Autodesk Inventor part; units mm, degrees
ref_plane "Work Plane1" through (-4, 0, 0) normal (1, 0, 0) x (0, 1, 0)
ref_plane "XZ Plane" through (0, 0, 0) normal (0, 1, 0) x (-1, 0, 0)
ref_plane "XY Plane" through (0, 0, 0) normal (0, 0, 1) x (1, 0, 0)
sketch "Sketch2" plane through (0, 0, 0) normal (0, 1, 0) x (-1, 0, 0)
  line L0 (-8, -4) -> (8, -4)
  line L1 (-8, 4) -> (8, 4)
  line L2 (-8, -4) -> (-8, 4)
  line L3 (8, 4) -> (8, -4)
  point P0 (0, 0)
  point P1 (0, 4)
  point P2 (-8, 0)
  dimension "d58" = 16
  dimension "d59" = 8
extrude "Extrusion1" add sketch "Sketch2" along normal blind 9.6
sketch "Sketch9" plane through (0, 0, 0) normal (0, -1, 0) x (1, 0, 0)
  line L0 (-8, 4) -> (8, 4)
  line L1 (-8, -4) -> (-8, 4)
  line L2 (-6.5, 2.5) -> (6.5, 2.5)
  line L3 (6.5, 2.5) -> (6.5, -2.5)
  line L4 (6.5, -2.5) -> (-6.5, -2.5)
  line L5 (-6.5, -2.5) -> (-6.5, 2.5)
  point P0 (0, 0)
  point P1 (0, 2.5)
  point P2 (-6.5, 0)
  dimension "d61" = 1.5
  dimension "d62" = 1.5
extrude "Extrusion4" cut sketch "Sketch9" against normal blind 8
sketch "Sketch11" plane through (-8, 0, 4) normal (0, 0, 1) x (1, 0, 0)
  line L0 (0, 0) -> (16, 0)
  line L1 (0, 9.6) -> (16, 9.6)
  line L2 (0, 0) -> (0, 9.6)
  line L3 (7.6, 8) -> (0.4, 8)
  line L4 (0.4, 8) -> (0.4, 5.6)
  arc A0 (0.4, 5.6) -> (7.6, 5.6) centre (4, 5.6) ccw
  line L5 (7.6, 5.6) -> (7.6, 8)
  point P0 (8, 0)
  point P1 (8, 9.6)
  dimension "d93" = 1.6
  dimension "d94" = 4
  dimension "d96" = 7.2
  dimension "d97" = 5.6
extrude "Extrusion5" add sketch "Sketch11" against normal blind 8
sketch "Sketch4" plane through (0, 9.6, 0) normal (0, 1, 0) x (1, 0, 0)
  circle A0 centre (-4, 0) radius 2.4
  circle A1 centre (-4, 0) radius 1.6
  line L0 (-8, 4) -> (-8, -4)
  point P0 (-8, 0)
  dimension "d13" = 4.8
  dimension "d57" = 3.2
  dimension "d69" = 4
extrude "Extrusion3" add sketch "Sketch4" along normal blind 1.6
sketch3d "Sketch12"
feature "LEGO_SM:1" [suppressed]
fillet "Fillet1" radius 0.1 1 edges at (-6.4, 11.2, 0)
pattern_linear "Rectangular Pattern2" count 2 spacing 8 along (1, 0, 0) of "Extrusion3", "Fillet1", "Extrusion5"
fillet "Fillet2" radius 0.1 8 edges at (-8, 9.6, 0) (-8, 4.8, 4) (0, 9.6, 4) (-8, 4.8, -4) (0, 9.6, -4) (8, 4.8, 4) (8, 9.6, 0) (8, 4.8, -4)
ref_plane "Work Plane1" through (-4, 0, 0) normal (1, 0, 0) x (0, 1, 0)
sketch "Sketch10" plane through (-4, 0, 0) normal (1, 0, 0) x (0, 1, 0)
  line L0 (0, -3.9) -> (0, 3.9)
  line L1 (0, 4) -> (9.5, 4)
  line L2 (9.5, -4) -> (0, -4)
  line L3 (5.6, 4) -> (5.6, -4)
  line L4 (5.6, -4) -> (8.8, -4)
  line L5 (8.8, -4) -> (8.8, -3.2)
  line L6 (8.8, -3.2) -> (8, -3.2)
  line L7 (8, -3.2) -> (8, 3.2)
  line L8 (8, 3.2) -> (8.8, 3.2)
  line L9 (8.8, 3.2) -> (8.8, 4)
  line L10 (8.8, 4) -> (5.6, 4)
  line L11 (8.8, 4) -> (9.5, 4)
  line L12 (9.5, -4) -> (8.8, -4)
  line L13 (9.5, -4) -> (9.5, 4)
  point P0 (0, 0)
  dimension "d75" = 5.6
  dimension "d76" = 0.8
  dimension "d77" = 4.8
  dimension "d78" = 6.4
revolve "Revolution1" cut sketch "Sketch10" angle 360 about axis through (-4, 5.6, 4) along (0, 0, -1) contours L1 L9 L8 L7 L6 L5 L2 L3
pattern_linear "Rectangular Pattern4" count 2 spacing 8 along (1, 0, 0) of "Revolution1"
equation "\"d58\" = 0.8 * knobs"
equation "\"d4\" = lh"
equation "\"d62\" = d61"
equation "\"d63\" = bd"
equation "\"d93\" = topthk"
equation "\"d96\" = tlad"
equation "\"d97\" = th"
equation "\"d13\" = kd"
equation "\"d57\" = rd"
equation "\"d69\" = 0.5 * lu"
equation "\"d20\" = knobh"
equation "\"d72\" = lu"
equation "\"d75\" = th"
equation "\"d76\" = tsl"
equation "\"d77\" = tpd"
equation "\"d78\" = tsd"
equation "\"d89\" = -0.5 * lu"
properties part number "32000-Black" material "ABS Plastic"
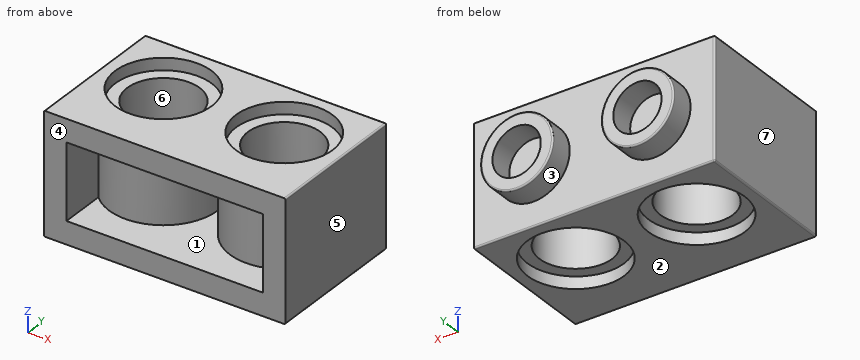
Part model, mm, in its own coordinate system. Face numbers are marked on the shaded views. A direction names the side the tool comes from. Coordinates: 2 decimals unless noted, no trailing zeros. Write each loop counter-clockwise with the first axis right and the second up, starting at its lowest first coordinate (ties: lowest second). Pieces come first, ordered by that corner, then holes. Notation, with made-up numbers: M 29,23.25 L 56,23.25 A32 ccw 56,57.25 Z; hole C -36,42 d11. An arc over 180 degrees is marked long. Return JSON: item names as keys, results as strings.
1. 3-axis set-ups, long thin cutter, end or side, ignore diameter. For the marked faces 1, 2 and 3: which of +Z, -Z, +X, -X, +Y, -Y reach the whole face in a straight line?
Determined:
{"face 1": "-Y", "face 2": "-Z, +X, -X, +Y, -Y", "face 3": "+Y"}
2. Flat gauge pins, fed straight in: pin 1 Ø3 at (x, y) = (5.5, 5) entering from -Z; pin 2 Ø2 at (x, z) = (-4.5, 0) entering from +Y. Where does each tip first touch, or does it go through?
Determined:
{"pin 1": "z = -3.2", "pin 2": "y = 9.6"}
3. Saw through at A-A, the plane z = 3. Write the cut outline in (x, y).
Determined:
{"outline": "M -8,0 L 8,0 L 8,9.5 A0.1 ccw 7.9,9.6 L -7.9,9.6 A0.1 ccw -8,9.5 Z; hole C -4,5.6 d4.8; hole C 4,5.6 d4.8"}
4. Probe L1, parallel to X at y = 10.15, z = 0; L2, parallel to X at y = 5.6, z = -3.55; L3, parallel to X at y = 5.6, z = 2. List the from-to ranges inside material, lowest first.
Determined:
{"L1": "-6.4 to -5.6, -2.4 to -1.6, 1.6 to 2.4, 5.6 to 6.4", "L2": "-8 to -7.2, -0.8 to 0.8, 7.2 to 8", "L3": "-8 to -6.4, -1.6 to -0.4, 0.4 to 1.6, 6.4 to 8"}
5. Pull direction X, two halves, no side cores. Call the marked faces 4, 5, 6 and 7: pulls with the +X half, pulls with the -X half, needs draft (parallel to the pull), parting line crosses it, or undercut.
Determined:
{"face 4": "needs draft", "face 5": "pulls with the +X half", "face 6": "undercut", "face 7": "pulls with the -X half"}
6. Saw through at C-C, the plane y = 5.25. Count the separate pieces of the cut face and the enclosed holes in it, then the cut area to 3 significant figures.
Determined:
{"separate pieces": "3", "enclosed holes": "1", "area": "42.7 mm²"}
